Part model, mm, in its own coordinate system. A direction names the side the tool comes from. Round coordinates to 2 decimals unless told otherwise and drop trailing zeros. Write each loop counter-clockwise with the first axis right and the second up, starting at its lowest first coordinate (ties: lowest second). Pieces come first, ordered by that corner, then holes.
```python
from build123d import *

# Parameters (mm, degrees)
SKETCH_1_R          = 22.5
EXTRUDE_1_DEPTH     = 5
SKETCH_2_R          = 17.5
EXTRUDE_2_DEPTH     = 85
EXTRUDE_3_DEPTH     = 2.5
SKETCH_4_R          = 2
CUT_EXTRUDE_1_DEPTH = 50


with BuildPart() as part:
    # Эскиз1 → Бобышка-Вытянуть1 (new body)
    with BuildSketch(Plane.XY):
        Circle(SKETCH_1_R)
    extrude(amount=EXTRUDE_1_DEPTH)

    # Эскиз2 → Бобышка-Вытянуть2 (add)
    with BuildSketch(Plane.XY.offset(5)):
        Circle(SKETCH_2_R)
    extrude(amount=EXTRUDE_2_DEPTH)

    # Эскиз3 → Бобышка-Вытянуть3 (add)
    with BuildSketch(Plane.XY.offset(90)):
        Polygon((10.606601718, 0), (0, 10.606601718), (-10.606601718, 0), (0, -10.606601718), align=None)
    extrude(amount=EXTRUDE_3_DEPTH)

    # Эскиз4 → Вырез-Вытянуть1 (cut)
    with BuildSketch(Plane.XY.offset(92.5)):
        Circle(SKETCH_4_R)
    extrude(amount=-CUT_EXTRUDE_1_DEPTH, mode=Mode.SUBTRACT)


solid = part.part
```
Q1. Drop flat-ended pins along their axis: pin 1 (10 mm diameter, centred on x = 4.5, z = 75.5, fed in from +Y); pin 2 (5 mm diameter, centred on x = -6.5, z = 79, fed in from +Y); pin 3 (8 mm diameter, centred on x = 9.5, z = 37.5, fed in from +Y); pin 4 (22.5 mm diameter, centred on x = -0.5, y = 11, fed in from +Z). Give the stop position or say it passes through.
Values follow:
pin 1: stops at y = 17.5
pin 2: stops at y = 17.04
pin 3: stops at y = 16.61
pin 4: stops at z = 92.5
Q2. Cut at A-A on y = 4.5. Write the cut outline in (x, z).
Values follow:
outline: (-22.05, 0) - (22.05, 0) - (22.05, 5) - (16.91, 5) - (16.91, 90) - (6.11, 90) - (6.11, 92.5) - (-6.11, 92.5) - (-6.11, 90) - (-16.91, 90) - (-16.91, 5) - (-22.05, 5) - close
Q3. Cut at B-B on z = 70. Write the cut outline in (x, y).
Values follow:
outline: circle Ø35 at (0, 0); hole circle Ø4 at (0, 0)
Q4. Which spindle directions (+Z, -Z, +X, -X, +Y, -Y) get a long thin tool onto all of the face, cutting with end or side? Do faces 1 (the flat face through (-5.378, -5.229, 91.232)), 2 (the flat face through (0, 0, 0)), 3 (the flat face through (5.229, -5.378, 91.232)), 4 (the flat face through (5.378, 5.229, 91.232)), 5 (the cylindrical face through (0, -2, 68)). Say none if no direction does.
Values follow:
face 1: +Z, -X, -Y
face 2: -Z, +X, -X, +Y, -Y
face 3: +Z, +X, -Y
face 4: +Z, +X, +Y
face 5: +Z
Q5. Wall check: L1, parallel to Z at x = -8, y = 15; L2, parallel to Z at x = -13, y = -17; L3, parallel to Y at x = -13.5, z = 51. Give the ranges that are in metal, low to high.
Values follow:
L1: z = 0 to 90
L2: z = 0 to 5
L3: y = -11.14 to 11.14
Q6. Cut at C-C on x = -16. Write the cut outline in (y, z).
Values follow:
outline: (-15.82, 0) - (15.82, 0) - (15.82, 5) - (7.09, 5) - (7.09, 90) - (-7.09, 90) - (-7.09, 5) - (-15.82, 5) - close
Q7. Cut at D-D on z = 12. Write the cut outline in (x, y), plus the area to 3 significant figures.
Values follow:
outline: circle Ø35 at (0, 0)
area: 962 mm2
Q8. Mould opens along Y. For faces 6 (the flat face through (-5.229, 5.378, 91.232)), 7 (the flat face through (12, -13, 5)), 8 (the flat face through (0, 0, 42.5)) say: +Y half, -Y half, draft (parallel to the pull), parting line (faces both ways), or undercut.
Values follow:
face 6: +Y half
face 7: draft
face 8: undercut
